Check sheet for the modelled part. Datum: model origin and axes. Units: mm. Face numbers are marked on the shaded views. A direction names the side the tool comes from. Coordinates: 2 decimals unless noted, no trailing zeros. Loops run counter-clockwise (first coordinate to the right, second up) from the corner with the lowest first, then second, coordinate; pieces in that order, holes last.
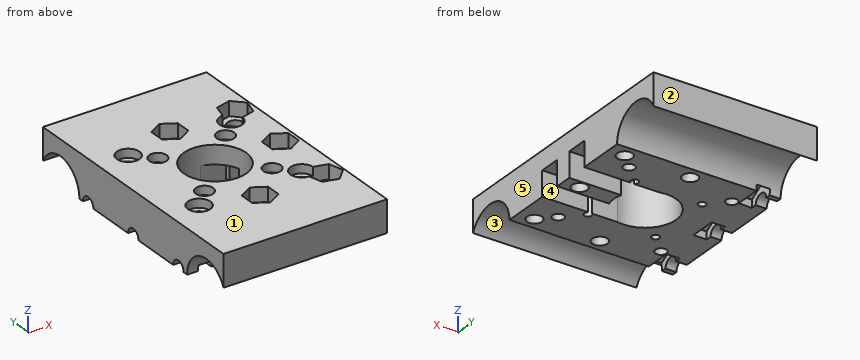
from build123d import *

# Parameters (mm, degrees)
SKETCH_W        = 75
SKETCH_H        = 120
PAD_DEPTH       = 20
POCKET_DEPTH    = 6.604
SKETCH002_R     = 3.5
POCKET001_DEPTH = 13.397
SKETCH003_R     = 5.2
SKETCH003_R_2   = 4
POCKET002_DEPTH = 4
SKETCH004_R     = 2.6
SKETCH004_R_2   = 1.75
POCKET003_DEPTH = 16.001
SKETCH005_R     = 14.3
POCKET004_DEPTH = 20.001
SKETCH006_W     = 10
SKETCH006_H     = 11.43
POCKET005_DEPTH = 37.5
SKETCH007_R     = 3.5
POCKET006_DEPTH = 5
POCKET007_DEPTH = 6.1
SKETCH009_R     = 12.7
POCKET008_DEPTH = 75.001


with BuildPart() as part:
    # Sketch → Pad (new body)
    with BuildSketch(Plane.XY):
        Rectangle(SKETCH_W, SKETCH_H)
    extrude(amount=PAD_DEPTH)

    # Sketch001 (on Face6 of Pad) → Pocket (cut)
    with BuildSketch(Plane.XY.offset(20)):
        Polygon((6.062178, 33.5), (0, 37), (-6.062178, 33.5), (-6.062178, 26.5), (0, 23), (6.062178, 26.5), align=None)
        Polygon((30, 7), (23.937822, 3.5), (23.937822, -3.5), (30, -7), (36.062178, -3.5), (36.062178, 3.5), align=None)
        Polygon((6.062178, -26.5), (0, -23), (-6.062178, -26.5), (-6.062178, -33.5), (0, -37), (6.062178, -33.5), align=None)
        Polygon((34.949747, 25.050253), (36.761481, 31.811733), (31.811733, 36.761481), (25.050253, 34.949747), (23.238519, 28.188267), (28.188267, 23.238519), align=None)
        Polygon((34.949747, -25.050253), (28.188267, -23.238519), (23.238519, -28.188267), (25.050253, -34.949747), (31.811733, -36.761481), (36.761481, -31.811733), align=None)
    extrude(amount=-POCKET_DEPTH, mode=Mode.SUBTRACT)

    # Sketch002 (on Face37 of Pocket) → Pocket001 (cut, through all)
    with BuildSketch(Plane.XY.offset(13.396)):
        with Locations((0, 30)):
            Circle(SKETCH002_R)
        with Locations((30, 30)):
            Circle(SKETCH002_R)
        with Locations((30, -30)):
            Circle(SKETCH002_R)
        with Locations((0, -30)):
            Circle(SKETCH002_R)
        with Locations((30, 0)):
            Circle(SKETCH002_R)
    extrude(amount=-POCKET001_DEPTH, mode=Mode.SUBTRACT)

    # Sketch003 (on Face5 of Pocket001) → Pocket002 (cut)
    with BuildSketch(Plane.XY.offset(20)):
        with Locations((-23.57, 23.57)):
            Circle(SKETCH003_R)
        with Locations((23.57, 23.57)):
            Circle(SKETCH003_R)
        with Locations((23.57, -23.57)):
            Circle(SKETCH003_R)
        with Locations((-23.57, -23.57)):
            Circle(SKETCH003_R)
        with Locations((-15.5, 15.5)):
            Circle(SKETCH003_R_2)
        with Locations((15.5, 15.5)):
            Circle(SKETCH003_R_2)
        with Locations((15.5, -15.5)):
            Circle(SKETCH003_R_2)
        with Locations((-15.5, -15.5)):
            Circle(SKETCH003_R_2)
    extrude(amount=-POCKET002_DEPTH, mode=Mode.SUBTRACT)

    # Sketch004 (on Face57 of Pocket002) → Pocket003 (cut, through all)
    with BuildSketch(Plane.XY.offset(16)):
        with Locations((-23.57, 23.57)):
            Circle(SKETCH004_R)
        with Locations((23.57, 23.57)):
            Circle(SKETCH004_R)
        with Locations((23.57, -23.57)):
            Circle(SKETCH004_R)
        with Locations((-23.57, -23.57)):
            Circle(SKETCH004_R)
        with Locations((-15.5, 15.5)):
            Circle(SKETCH004_R_2)
        with Locations((15.5, 15.5)):
            Circle(SKETCH004_R_2)
        with Locations((-15.5, -15.5)):
            Circle(SKETCH004_R_2)
        with Locations((15.5, -15.5)):
            Circle(SKETCH004_R_2)
    extrude(amount=-POCKET003_DEPTH, mode=Mode.SUBTRACT)

    # Sketch005 (on Face5 of Pocket003) → Pocket004 (cut, through all)
    with BuildSketch(Plane.XY.offset(20)):
        Circle(SKETCH005_R)
    extrude(amount=-POCKET004_DEPTH, mode=Mode.SUBTRACT)

    # Sketch006 (on Face3 of Pocket004) → Pocket005 (cut)
    with BuildSketch(Plane.YZ.offset(37.5)):
        with Locations((-9, 5.715)):
            Rectangle(SKETCH006_W, SKETCH006_H)
        with Locations((9, 5.715)):
            Rectangle(SKETCH006_W, SKETCH006_H)
    extrude(amount=-POCKET005_DEPTH, mode=Mode.SUBTRACT)

    # Sketch007 (on Face2 of Pocket005) → Pocket006 (cut)
    with BuildSketch(Plane(origin=(-37.5, 0, 0), x_dir=(0, -1, 0), z_dir=(-1, 0, 0))):
        with Locations((-30, 0)):
            Circle(SKETCH007_R)
        Circle(SKETCH007_R)
        with Locations((30, 0)):
            Circle(SKETCH007_R)
    extrude(amount=-POCKET006_DEPTH, mode=Mode.SUBTRACT)

    # Sketch008 (on Face22 of Pocket006) → Pocket007 (cut)
    with BuildSketch(Plane(origin=(-32.5, 0, 0), x_dir=(0, -1, 0), z_dir=(-1, 0, 0))):
        Polygon((-36.062178, -3.5), (-30, -7), (-23.937822, -3.5), (-23.937822, 3.5), (-30, 7), (-36.062178, 3.5), align=None)
        Polygon((-6.062178, -3.5), (0, -7), (6.062178, -3.5), (6.062178, 3.5), (0, 7), (-6.062178, 3.5), align=None)
        Polygon((36.062178, 3.5), (30, 7), (23.937822, 3.5), (23.937822, -3.5), (30, -7), (36.062178, -3.5), align=None)
    extrude(amount=-POCKET007_DEPTH, mode=Mode.SUBTRACT)

    # Sketch009 (on Face3 of Pocket007) → Pocket008 (cut, through all)
    with BuildSketch(Plane.YZ.offset(37.5)):
        with Locations((-48.5, 0)):
            Circle(SKETCH009_R)
        with Locations((48.5, 0)):
            Circle(SKETCH009_R)
    extrude(amount=-POCKET008_DEPTH, mode=Mode.SUBTRACT)


solid = part.part
(1) Section check C-C, the plane x = -9.5. Enter the section's corners in (y, z).
(2) Draft check along Y on the marked faces 1, 2 and 3. Enter one of: pulls with the +Y half, pulls with the -Y half, needs draft (parallel to the pull), parting line crosses it, or undercut.
(3) Section check A-A, the plane x = -23.57. Enter the section's corners in (y, z).
(4) Set-up check for the marked faces 4 and 5: record each of +Z, -Z, +X, -X, +Y, -Y from which the full face is reachable in a straight line by a thin tool's end or side.
(5) Section check B-B, the plane y = -15.5. Enter the section's corners in (x, z).
(6) Gauge pin test, flat ends, axial feed: P1, Ø6.5, axis at x = 0, y = 30, coming from the -Z side; P2, Ø7, axis at x = 23.57, y = -23.57, coming from the +Z side; P3, Ø3, axis at x = -29.5, z = 2, coming from the -Y side; P4, Ø1, axis at x = -17.5, z = 4, coming from the +Y side. Record the tip position at first contact, or that the pin passes through.
(7) Scan lines: line 1 along X through (y, z) = (1.5, 10.75); line 2 along X through (y, z) = (-12, 18.5); line 3 along Y through (x, z) = (30, 3.5). Record each from-to range of solid material in increasing order.
(8) Section check D-D, the plane z = 17.25. Count the separate pieces of the cut face and the enclosed holes in it, plus the area to 3 significant figures.
Determined:
1. outline: (-60, 5.39) arc R12.7 cw to (-35.8, 0) - (-10.69, 0) - (-10.69, 20) - (-60, 20) - close; (10.69, 0) - (35.8, 0) arc R12.7 cw to (60, 5.39) - (60, 20) - (10.69, 20) - close
2. face 1: needs draft
2. face 2: pulls with the +Y half
2. face 3: undercut
3. outline: (-60, 5.39) arc R12.7 cw to (-35.8, 0) - (-26.17, 0) - (-26.17, 16) - (-28.77, 16) - (-28.77, 20) - (-60, 20) - close; (-20.97, 0) - (20.97, 0) - (20.97, 16) - (18.37, 16) - (18.37, 20) - (-18.37, 20) - (-18.37, 16) - (-20.97, 16) - close; (26.17, 0) - (35.8, 0) arc R12.7 cw to (60, 5.39) - (60, 20) - (28.77, 20) - (28.77, 16) - (26.17, 16) - close
4. face 4: -Z, +X
4. face 5: +Z, -Z, +X, +Y, -Y
5. outline: (-37.5, 0) - (-17.25, 0) - (-17.25, 16) - (-19.5, 16) - (-19.5, 20) - (-37.5, 20) - close; (-13.75, 0) - (13.75, 0) - (13.75, 16) - (11.5, 16) - (11.5, 20) - (-11.5, 20) - (-11.5, 16) - (-13.75, 16) - close; (17.25, 0) - (37.5, 0) - (37.5, 20) - (19.5, 20) - (19.5, 16) - (17.25, 16) - close
6. P1: passes through
6. P2: stops at z = 16
6. P3: stops at y = -36.29
6. P4: stops at y = 36.62
7. line 1: x = -37.5 to -14.22, 14.22 to 26.84, 33.16 to 37.5
7. line 2: x = -37.5 to -17.44, -13.56 to -7.78, 7.78 to 13.56, 17.44 to 37.5
7. line 3: y = -36.29 to -33.5, -26.5 to -14, -4 to -3.5, 3.5 to 4, 14 to 26.5, 33.5 to 36.29
8. separate pieces: 1
8. enclosed holes: 12
8. area: 7,210 mm2
